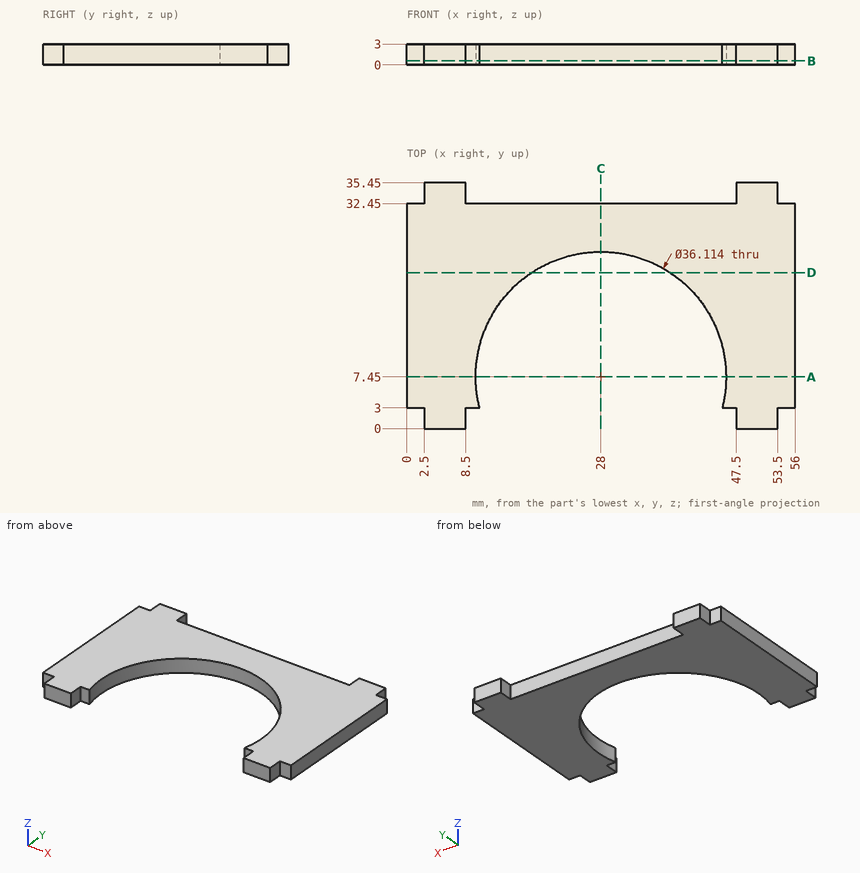
Geometry check sheet. Reference: drawing and pictorial views, mm from the part's lowest x, y, z. Coordinates: 2 decimals unless noted, no trailing zeros. Loops run counter-clockwise (first coordinate to the right, second up) from the corner with the lowest first, then second, coordinate; pieces in that order, holes last. Notation, with made-up numbers: (-35, -26) - (-29, -26) arc R23 ccw to (-29, -1) - close; hole circle Ø8 at (36, 64.5). An arc over 180 degrees is marked (long way). Return JSON: item names as keys, results as strings.
1. Section check A-A, the plane y = 7.45. Record the boundary of the cut face in (x, z).
Established:
{"outline": "(0, 0) - (9.94, 0) - (9.94, 3) - (0, 3) - close; (46.06, 0) - (56, 0) - (56, 3) - (46.06, 3) - close"}
2. Section check D-D, the plane y = 22.5. Record the boundary of the cut face in (x, z).
Established:
{"outline": "(0, 0) - (18.02, 0) - (18.02, 3) - (0, 3) - close; (37.98, 0) - (56, 0) - (56, 3) - (37.98, 3) - close"}
3. Go/stop test with flat-tipped pins: pin 1 (1.5 mm diameter, centred on y = 1, z = 1, fed in from -X); pin 2 (1.5 mm diameter, centred on y = 34.5, z = 1, fed in from +X); pin 3 (0.8 mm diameter, centred on x = 1.5, z = 1.5, fed in from +Y). Record where each tip stops, or that it passes through.
Established:
{"pin 1": "stops at x = 2.5", "pin 2": "stops at x = 53.5", "pin 3": "stops at y = 32.45"}
4. Section check C-C, the plane x = 28. Record the boundary of the cut face in (y, z), then the cut area to 3 significant figures.
Established:
{"outline": "(25.51, 0) - (32.45, 0) - (32.45, 3) - (25.51, 3) - close", "area": "20.8 mm2"}
5. Thickness scan on L1, parallel to X at y = 7.45, z = 1.35; L2, parallel to X at y = 21, z = 2.55 (1 decimal); L3, parallel to Y at x = 39, z = 0.9. Record the ranges inside material, lowest first.
Established:
{"L1": "x = 0 to 9.94, 46.06 to 56", "L2": "x = 0 to 16.1, 39.9 to 56", "L3": "y = 21.77 to 32.45"}
6. Section check B-B, the plane z = 0.55. Record the boundary of the cut face in (x, y).
Established:
{"outline": "(0, 3) - (2.5, 3) - (2.5, 0) - (8.5, 0) - (8.5, 3) - (10.5, 3) arc R18.06 cw (long way) to (45.5, 3) - (47.5, 3) - (47.5, 0) - (53.5, 0) - (53.5, 3) - (56, 3) - (56, 32.45) - (53.5, 32.45) - (53.5, 35.45) - (47.5, 35.45) - (47.5, 32.45) - (8.5, 32.45) - (8.5, 35.45) - (2.5, 35.45) - (2.5, 32.45) - (0, 32.45) - close"}
